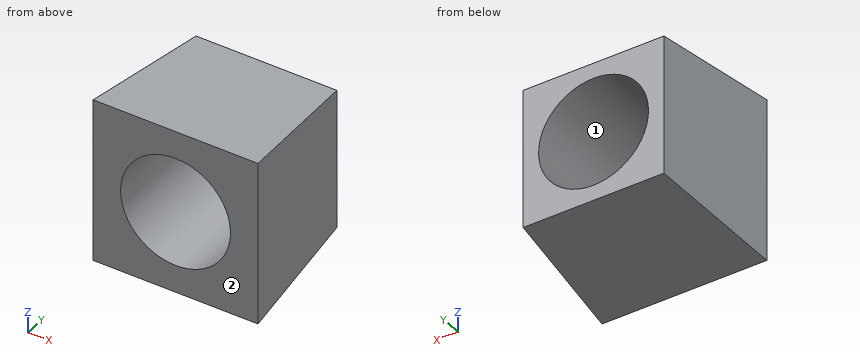
```python
from build123d import *

# Parameters (mm, degrees)
ESQUISSE1_W             = 30
ESQUISSE1_H             = 30
EXTRUSION1_DEPTH        = 25
EXTRUSION1_TAPER        = 5
ESQUISSE2_R             = 10
ENL_V_MAT_EXTRU_1_DEPTH = 26.0000001


with BuildPart() as part:
    # Esquisse1 → Extrusion1 (new body)
    with BuildSketch(Plane(origin=(0, 0, 0), x_dir=(1, 0, 0), z_dir=(0, 1, 0))):
        with Locations((15, 15)):
            Rectangle(ESQUISSE1_W, ESQUISSE1_H)
    extrude(amount=EXTRUSION1_DEPTH, taper=EXTRUSION1_TAPER)

    # Esquisse2 → Enlèv. mat.-Extru.1 (cut, through all)
    with BuildSketch(Plane.XZ):
        with Locations((15, -15)):
            Circle(ESQUISSE2_R)
    extrude(amount=-ENL_V_MAT_EXTRU_1_DEPTH, mode=Mode.SUBTRACT)


solid = part.part
```
The listing builds one solid part. Answer for the finished solid, in the listing's coordinates (mm). Face numbers are marked on the shaded views. Give positions to 0.01 mm unless a question says otherwise; leave off trailing zeros. Answer in a Markdown table with one row per item. Add a question column.
Q1. For a pull along X with two mould halves and no side action, classify the marked faces 1 and 2 as released by +X, released by -X, zero draft, split by the parting line, or undercut.
Q2. Find the intervals of material crossed by line 1 along Z through (x, y) = (17, 9.5); line 2 along Z through (x, y) = (15, 7.25); line 3 along X through (y, z) = (21, -17), in increasing order. Write a range as [from, to].
Q3. Given P1, Ø1.5, axis at y = 22, z = -26.5, coming from the +X side; P2, Ø2, axis at y = 4, z = -12.5, coming from the -X side; P3, Ø1, axis at x = 19.5, z = -3.5, coming from the -Y side; P4, Ø1, axis at x = 8, y = 15.5, coming from the +Z side, each flat-ended and moving along its own axis, determine where each tip first touches the part or whether it passes through.
Determined:
| question | item | result |
|---|---|---|
| 1 | face 1 | undercut |
| 1 | face 2 | zero draft |
| 2 | line 1 | z = [-29.17, -24.8], [-5.2, -0.83] |
| 2 | line 2 | z = [-29.37, -25], [-5, -0.63] |
| 2 | line 3 | x = [1.84, 5.2], [24.8, 28.16] |
| 3 | P1 | stops at x = 28.14 |
| 3 | P2 | stops at x = 0.26 |
| 3 | P3 | stops at y = 0 |
| 3 | P4 | stops at z = -1.31 |
